Read the model definition and answer for the solid it produces. Units are mm, in the model's axes. Face numbers are marked on the shaded views. A direction names the side the tool comes from. Give positions to 0.01 mm unless a question says otherwise; leave off trailing zeros. Loops run counter-clockwise (first coordinate to the right, second up) from the corner with the lowest first, then second, coordinate; pieces in that order, holes last.
(1) Find section C-C, the plane z = -8. Write down the section's boundary in (x, y), then the cut area to 3 significant figures.
(2) Find section D-D, the plane y = 15.5. Write down the section's boundary in (x, z).
(3) This flat-tipped pin is pushed along its axis until it touches: P1, Ø1.9, axis at x = 15.5, y = -15, coming from the +Z side. Where does it stop, or does it pass through?
(4) Determine the mould class of the marked faces 3, 4, 5 and 6 for opening direction X: pulls with the +X half, pulls with the -X half, needs draft (parallel to the pull), parting line crosses it, or undercut.
(5) Straight lines are drawn through the part: probe 1 along Y at (x, z) = (-15.5, -2.5); probe 2 along X at (y, z) = (19.5, -4.5); probe 3 along X at (y, z) = (18, -1.5). For each, find the intervals that lie inside material, in ascending order.
(6) Which of the six approach directions +Z, -Z, +X, -X, +Y, -Y give full straight-line access (tool end or side, diameter ignored) to the marked faces 1 and 2?
(7) Find section A-A, the plane y = 3.5. Write down the section's boundary in (x, z).
(8) Find section B-B, the plane x = 0. Write down the section's boundary in (y, z), then the cut area to 3 significant figures.
Solid Edge part; units mm, degrees
sketch "Sketch1" plane through (0, 0, 0) normal (0, 0, 1) x (1, 0, 0)
  line L0 (-25, 22) -> (25, 22)
  line L1 (25, 22) -> (25, -22)
  line L2 (25, -22) -> (-25, -22)
  line L3 (-25, -22) -> (-25, 22)
  line L4 (-14.2979, 16.7021) -> (-10.7624, 13.1665)
  arc A0 (-13.1665, 10.7624) -> (-10.7624, 13.1665) centre (-11.9645, 11.9645) ccw
  line L5 (-16.7021, 14.2979) -> (-13.1665, 10.7624)
  arc A1 (-16.7021, 14.2979) -> (-14.2979, 16.7021) centre (-15.5, 15.5) cw
  line L6 (14.2979, 16.7021) -> (10.7624, 13.1665)
  arc A2 (10.7624, 13.1665) -> (13.1665, 10.7624) centre (11.9645, 11.9645) ccw
  line L7 (16.7021, 14.2979) -> (13.1665, 10.7624)
  arc A3 (16.7021, 14.2979) -> (14.2979, 16.7021) centre (15.5, 15.5) ccw
  line L8 (16.7021, -14.2979) -> (13.1665, -10.7624)
  arc A4 (10.7624, -13.1665) -> (13.1665, -10.7624) centre (11.9645, -11.9645) cw
  line L9 (14.2979, -16.7021) -> (10.7624, -13.1665)
  arc A5 (14.2979, -16.7021) -> (16.7021, -14.2979) centre (15.5, -15.5) ccw
  line L10 (-14.2979, -16.7021) -> (-10.8303, -13.2345)
  arc A6 (-13.1705, -10.7663) -> (-10.8303, -13.2345) centre (-12.0333, -12.0316) cw
  line L11 (-13.1705, -10.7663) -> (-16.7021, -14.2979)
  arc A7 (-16.7021, -14.2979) -> (-14.2979, -16.7021) centre (-15.5, -15.5) ccw
  circle A8 centre (0, 0) radius 12.5
  dimension "D1" = 25
  dimension "D2" = 25
extrude "Protrusion1" add sketch "Sketch1" against normal blind 10
sketch "Sketch2" plane through (0, 0, 0) normal (0, 0, 1) x (0, -1, 0)
  circle A0 centre (-15.5, 15.5) radius 3.2
  circle A1 centre (15.5, 15.5) radius 3.2
  circle A2 centre (15.5, -15.5) radius 3.2
  circle A3 centre (-15.5, -15.5) radius 3.2
extrude "ExtrudedCutout_1" cut sketch "Sketch2" against normal blind 4
sketch "Sketch3" plane through (0, -22, -3.5) normal (0, -1, 0) x (1, 0, 0)
  line L0 (19.0832, -0.0858) -> (20.4974, 1.3284)
  line L1 (20.4974, 1.3284) -> (21.9116, -0.0858)
  arc A0 (21.9116, -0.0858) -> (19.0832, -0.0858) centre (20.4974, -1.5) cw
  line L2 (-22.2076, -0.0858) -> (-20.7957, 1.3261)
  line L3 (-20.7957, 1.3261) -> (-19.462, -0.0076)
  arc A1 (-19.462, -0.0076) -> (-22.2076, -0.0858) centre (-20.7934, -1.5) cw
  dimension "D1" = 20.7934
extrude "ExtrudedCutout_2" cut sketch "Sketch3" against normal blind 168.7822
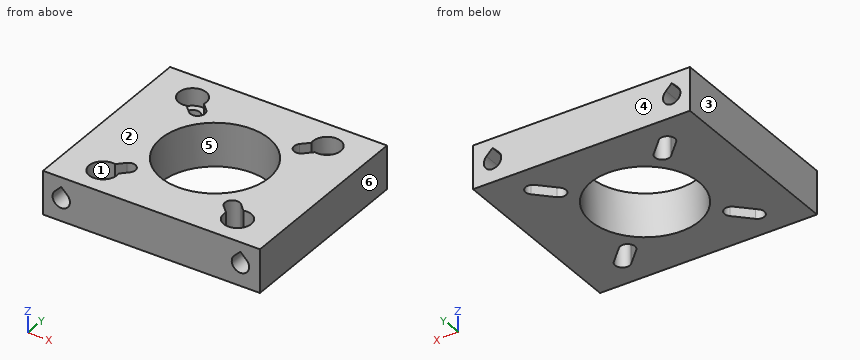
Entries:
1. outline: (-25, -22) - (25, -22) - (25, 22) - (-25, 22) - close; hole (-16.7, -14.3) arc R1.7 ccw to (-14.3, -16.7) - (-10.83, -13.23) arc R1.7 ccw to (-13.17, -10.77) - close; hole (-16.7, 14.3) - (-13.17, 10.76) arc R1.7 ccw to (-10.76, 13.17) - (-14.3, 16.7) arc R1.7 ccw to start; hole circle Ø25 at (0, 0); hole (10.76, -13.17) - (14.3, -16.7) arc R1.7 ccw to (16.7, -14.3) - (13.17, -10.76) arc R1.7 ccw to start; hole (10.76, 13.17) arc R1.7 ccw to (13.17, 10.76) - (16.7, 14.3) arc R1.7 ccw to (14.3, 16.7) - close
1. area: 1,610 mm2
2. outline: (-25, -10) - (-17.2, -10) - (-17.2, -4) - (-18.7, -4) - (-18.7, 0) - (-25, 0) - close; (-13.1, -10) - (13.1, -10) - (13.1, -4) - (12.3, -4) - (12.3, 0) - (-12.3, 0) - (-12.3, -4) - (-13.1, -4) - close; (17.2, -10) - (25, -10) - (25, 0) - (18.7, 0) - (18.7, -4) - (17.2, -4) - close; hole (-22.21, -3.59) arc R2 ccw (long way) to (-19.46, -3.51) - (-20.8, -2.17) - close; hole (19.08, -3.59) arc R2 ccw (long way) to (21.91, -3.59) - (20.5, -2.17) - close
3. P1: passes through
4. face 3: pulls with the -X half
4. face 4: needs draft
4. face 5: undercut
4. face 6: pulls with the +X half
5. probe 1: y = -22 to -18.7, -12.3 to 12.3, 18.7 to 22
5. probe 2: x = -25 to -22.73, -18.86 to 18.56, 22.43 to 25
5. probe 3: x = -25 to -17.5, -13.5 to 13.5, 17.5 to 25
6. face 1: +Z
6. face 2: +Z, +X, -X, +Y, -Y
7. outline: (-25, -10) - (-12, -10) - (-12, 0) - (-25, 0) - close; (12, -10) - (25, -10) - (25, 0) - (12, 0) - close; hole (-22.21, -3.59) arc R2 ccw (long way) to (-19.46, -3.51) - (-20.8, -2.17) - close; hole (19.08, -3.59) arc R2 ccw (long way) to (21.91, -3.59) - (20.5, -2.17) - close
8. outline: (-22, -10) - (-12.5, -10) - (-12.5, 0) - (-22, 0) - close; (12.5, -10) - (22, -10) - (22, 0) - (12.5, 0) - close
8. area: 190 mm2
